from build123d import *

# Parameters (mm, degrees)
CIRCLE001_R            = 2.5
EXTRUDE009_DEPTH       = 1.5
EXTRUDE010_DEPTH       = 1.5
CUT001_PLACEMENT_ANGLE = 90


with BuildPart() as extrude009:
    # Circle001 → Extrude009 (new body)
    with BuildSketch(Plane(origin=(10, 0, 0), x_dir=(1, 0, 0), z_dir=(0, 0, -1))):
        Circle(CIRCLE001_R)
    extrude(amount=-EXTRUDE009_DEPTH)


with BuildPart() as ecrou:
    # Polygon001 → Extrude010 (new body)
    with BuildSketch(Plane(origin=(10, 0, 0), x_dir=(1, 0, 0), z_dir=(0, 0, 1))):
        with BuildLine():
            Line((2.453739, 3.75), (4.474465, 0.25))
            ThreePointArc((4.474465, 0.25), (4.541452, 0), (4.474465, -0.25))
            Line((4.474465, -0.25), (2.453739, -3.75))
            ThreePointArc((2.453739, -3.75), (2.270726, -3.933013), (2.020726, -4))
            Line((2.020726, -4), (-2.020726, -4))
            ThreePointArc((-2.020726, -4), (-2.270726, -3.933013), (-2.453739, -3.75))
            Line((-2.453739, -3.75), (-4.474465, -0.25))
            ThreePointArc((-4.474465, -0.25), (-4.541452, 0), (-4.474465, 0.25))
            Line((-4.474465, 0.25), (-2.453739, 3.75))
            ThreePointArc((-2.453739, 3.75), (-2.270726, 3.933013), (-2.020726, 4))
            Line((-2.020726, 4), (2.020726, 4))
            ThreePointArc((2.020726, 4), (2.270726, 3.933013), (2.453739, 3.75))
        make_face()
    extrude(amount=EXTRUDE010_DEPTH)

    # Cut001: cut Extrude009
    add(extrude009.part, mode=Mode.SUBTRACT)


with BuildPart() as ecrou_1:
    # Cut001 placement: moved
    add(ecrou.part.moved(Location((25, 40, 9))).rotate(Axis((25, 40, 9), (0, 0, 1)), CUT001_PLACEMENT_ANGLE))


solid = ecrou_1.part
CAD build for the part. Positions are in the model's coordinates, mm. Round coordinates to 2 decimals unless told otherwise and drop trailing zeros. Loops run counter-clockwise (first coordinate to the right, second up) from the corner with the lowest first, then second, coordinate; pieces in that order, holes last. Notation, with made-up numbers: (-31.75, 42) - (-5.75, 42) arc R19 ccw to (-5.75, 79) - close; hole circle Ø9 at (42, 71). An arc over 180 degrees is marked (long way). Put each result on its own line as item: value.
1. Two-plate mould, pull along Y, no slides. Class faces 1 (the flat face through (26.976, 53.478, 9.74)), 2 (the flat face through (27, 48, 10.5)), 3 (the cylindrical face through (27.11, 51.34, 9.74)): released by +Y, released by -Y, zero draft, split by the parting line, or undercut.
Geometry check:
face 1: released by +Y
face 2: zero draft
face 3: undercut
2. Wall check: line 1 (X direction, y = 50, z = 10.2); line 2 (Y direction, x = 23, z = 9.1); line 3 (X direction, y = 47.75, z = 10.2). Give the ranges that are in metal, low to high.
Geometry check:
line 1: 21 to 22.5, 27.5 to 29
line 2: 46.54 to 48.5, 51.5 to 53.46
line 3: 21.06 to 23.91, 26.09 to 28.94
3. Slice it at A-A on y = 50. List the corners of the cut face in (x, z), and give its area (3 significant figures).
Geometry check:
outline: (21, 9) - (22.5, 9) - (22.5, 10.5) - (21, 10.5) - close; (27.5, 9) - (29, 9) - (29, 10.5) - (27.5, 10.5) - close
area: 4.50 mm²
4. Slice it at C-C on x = 25. List the corners of the cut face in (y, z).
Geometry check:
outline: (45.46, 9) - (47.5, 9) - (47.5, 10.5) - (45.46, 10.5) - close; (52.5, 9) - (54.54, 9) - (54.54, 10.5) - (52.5, 10.5) - close
5. Slice it at B-B on z = 9.6. List the corners of the cut face in (x, y), and give its area (3 significant figures).
Geometry check:
outline: (21, 47.98) arc R0.5 ccw to (21.25, 47.55) - (24.75, 45.53) arc R0.5 ccw to (25.25, 45.53) - (28.75, 47.55) arc R0.5 ccw to (29, 47.98) - (29, 52.02) arc R0.5 ccw to (28.75, 52.45) - (25.25, 54.47) arc R0.5 ccw to (24.75, 54.47) - (21.25, 52.45) arc R0.5 ccw to (21, 52.02) - close; hole circle Ø5 at (25, 50)
area: 35.7 mm²
6. Slice it at D-D on y = 52.75. List the corners of the cut face in (x, z).
Geometry check:
outline: (21.76, 9) - (28.24, 9) - (28.24, 10.5) - (21.76, 10.5) - close
